```python
from build123d import *

# Parameters (mm, degrees)
F0_R          = 25.4
F1_DEPTH      = 457.2
F2_W          = 57.15
F2_H          = 76.2
F2_H_2        = 152.4
F2_H_3        = 79.4389369488
F3_DEPTH      = 28.576
F3_DEPTH_BACK = 28.576
F4_W          = 3.175
F4_H          = 457.2
F5_DEPTH      = 742.95


with BuildPart() as f1:
    # F0 (on Top) → F1 (new body)
    with BuildSketch(Plane.XY):
        with BuildLine():
            Line((-28.575, 800.1), (-28.575, 0))
            ThreePointArc((-28.575, 0), (27.7699083992, -6.7351920908), (-25.4, 13.0908603613))
            Line((-25.4, 13.0908603613), (-25.4, 800.1))
            Line((-25.4, 800.1), (-28.575, 800.1))
        make_face()
        Circle(F0_R, mode=Mode.SUBTRACT)
    extrude(amount=F1_DEPTH)

    # F2 (on Right) → F3 (cut, two sides)
    with BuildSketch(Plane.YZ) as f3_sk:
        with Locations((0, 38.1)):
            Rectangle(F2_W, F2_H)
        with Locations((0, 228.6)):
            Rectangle(F2_W, F2_H_2)
        with Locations((0, 420.7194684744)):
            Rectangle(F2_W, F2_H_3)
    extrude(amount=-F3_DEPTH, mode=Mode.SUBTRACT)
    extrude(f3_sk.sketch, amount=F3_DEPTH_BACK, mode=Mode.SUBTRACT)

    # F4 (on face) → F5 (join)
    with BuildSketch(Plane(origin=(0, 800.1, 0), x_dir=(-1, 0, 0), z_dir=(0, 1, 0))):
        with Locations((26.9875, 228.6)):
            Rectangle(F4_W, F4_H)
    extrude(amount=F5_DEPTH)


solid = f1.part
```
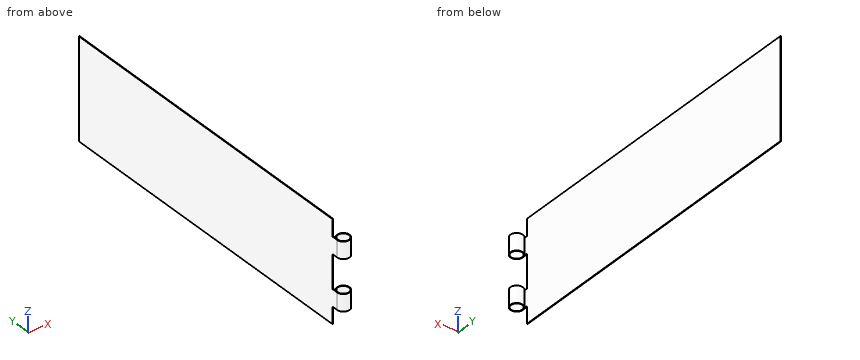
Geometry check sheet. Reference: the model listing, model coordinates, mm. Give positions to 0.01 mm unless a question says otherwise; leave off trailing zeros. Order: outer loops, then holes, each group sorted by start corner. A loop starts at its lowest first (then second) coordinate and runs counter-clockwise, first axis right, second up.
1. Gauge pin test, flat ends, axial feed: pin 1 Ø1.6 at (x, z) = (-27.5, 418.5) entering from -Y (3 decimals); pin 2 Ø8 at (x, z) = (-8, 353.5) entering from -Y; pin 3 Ø3 at (y, z) = (1198.5, 107.5) entering from +X. Record the tip position at first contact, or that the pin passes through.
2. Thickness scan on L1, parallel to Y at x = 0, z = 128 (3 decimals); L2, parallel to X at y = 1462.5, z = 432.5 (3 decimals); L3, parallel to Y at x = -7, z = 319. Record the ranges inside material, lowest first.
3. Section check C-C, the plane z = 426. Enter the section's corners in (x, y) (3 decimals), and give its area (3 significant figures).
4. Section check A-A, the plane x = 0. Enter the section's corners in (y, z) (3 decimals), and give its area (3 significant figures).
5. Section check B-B, the plane y = 871. Enter the section's corners in (x, z) (3 decimals), and give its area (3 significant figures).
Values follow:
1. pin 1: stops at y = 28.575
1. pin 2: stops at y = -28.29
1. pin 3: stops at x = -25.4
2. L1: y = -28.575 to -25.4, 25.4 to 28.575
2. L2: x = -28.575 to -25.4
2. L3: y = -27.7 to -24.42, 24.42 to 27.7
3. outline: (-28.575, 28.575) - (-25.4, 28.575) - (-25.4, 1543.05) - (-28.575, 1543.05) - close
3. area: 4,810 mm2
4. outline: (-28.575, 76.2) - (-25.4, 76.2) - (-25.4, 152.4) - (-28.575, 152.4) - close; (-28.575, 304.8) - (-25.4, 304.8) - (-25.4, 381) - (-28.575, 381) - close; (25.4, 76.2) - (28.575, 76.2) - (28.575, 152.4) - (25.4, 152.4) - close; (25.4, 304.8) - (28.575, 304.8) - (28.575, 381) - (25.4, 381) - close
4. area: 968 mm2
5. outline: (-28.575, 0) - (-25.4, 0) - (-25.4, 457.2) - (-28.575, 457.2) - close
5. area: 1,450 mm2
